```python
from build123d import *

# Parameters (mm, degrees)
F0_W     = 21.082
F0_H     = 12.7
F1_DEPTH = 5.08
F2_R     = 2.5019
F3_DEPTH = 5.08
F4_R     = 0.127


with BuildPart() as f1:
    # F0 (on Top) → F1 (new body)
    with BuildSketch(Plane.XY):
        Rectangle(F0_W, F0_H)
        with BuildLine():
            Line((-10.541, -6.35), (-10.541, 6.35))
            ThreePointArc((-10.541, 6.35), (-16.891, 0), (-10.541, -6.35))
        make_face()
        with BuildLine():
            ThreePointArc((10.541, -6.35), (16.891, 0), (10.541, 6.35))
            Line((10.541, 6.35), (10.541, -6.35))
        make_face()
    extrude(amount=F1_DEPTH)

    # F2 (on face) → F3 (join)
    with BuildSketch(Plane.XY.offset(5.08)):
        with Locations((-10.541, 0)):
            Circle(F2_R)
        with Locations((10.541, 0)):
            Circle(F2_R)
    extrude(amount=F3_DEPTH)

    # F4
    f4_edges = [f1.edges().sort_by_distance(p)[0] for p in [
        (-13.0429, 0, 10.16),
        (8.0391, 0, 10.16),
    ]]
    fillet(f4_edges, radius=F4_R)


solid = f1.part
```
Geometry check sheet. Reference: the model listing, model coordinates, mm. A direction names the side the tool comes from. Give positions to 0.01 mm unless a question says otherwise; leave off trailing zeros. Write each loop counter-clockwise with the first axis right and the second up, starting at its lowest first coordinate (ties: lowest second). Pieces come first, ordered by that corner, then holes. Notation, with made-up numbers: (40, -32.5) -> (69, -32.5) arc R9 cw to (69, -27.5) -> close; hole circle Ø10 at (76, 54). An arc over 180 degrees is marked (long way). Use one line per item in the form item = value.
Item 1: Sectioned sample at D-D on z = 2. Enter the section's corners in (x, y).
Results list:
outline = (-10.54, -6.35) -> (10.54, -6.35) arc R6.35 ccw to (10.54, 6.35) -> (-10.54, 6.35) arc R6.35 ccw to start
Item 2: Depth check by flat-ended pin: pin 1 Ø2 at (x, y) = (-4.5, -3) entering from +Z; pin 2 Ø1 at (y, z) = (5, 1) entering from -X. Enter the tip coordinate at first touch or a pass-through.
Results list:
pin_1 = 5.08
pin_2 = -15.02
Item 3: Access from +Z, -Z, +X, -X, +Y, -Y to the whole of each face (thin tool, end or side, straight path). Record for faces 1 (the cylindrical face through (8.04, 0.11, 7.52)), 2 (the flat face through (0, 0, 0)).
Results list:
face_1 = +Z
face_2 = -Z, +X, -X, +Y, -Y
Item 4: Mould release check, pull along X, two halves, no side actions. Record for faces 3 (the cylindrical face through (16.89, -0.14, 2.5)), 4 (the flat face through (0, 0, 5.08)), 5 (the cylindrical face through (-13.04, 0.11, 7.52)), 6 (the flat face through (0, 6.35, 3)): released by +X, released by -X, zero draft, split by the parting line, or undercut.
Results list:
face_3 = released by +X
face_4 = undercut
face_5 = undercut
face_6 = zero draft
Item 5: Sectioned sample at C-C on x = -5.5. Enter the section's corners in (y, z), plus the area to 3 significant figures.
Results list:
outline = (-6.35, 0) -> (6.35, 0) -> (6.35, 5.08) -> (-6.35, 5.08) -> close
area = 64.5 mm2
Item 6: Sectioned sample at A-A on y = 0. Enter the section's corners in (x, z), plus the area to 3 significant figures.
Results list:
outline = (-16.89, 0) -> (16.89, 0) -> (16.89, 5.08) -> (13.04, 5.08) -> (13.04, 10.03) arc R0.13 ccw to (12.92, 10.16) -> (8.17, 10.16) arc R0.13 ccw to (8.04, 10.03) -> (8.04, 5.08) -> (-8.04, 5.08) -> (-8.04, 10.03) arc R0.13 ccw to (-8.17, 10.16) -> (-12.92, 10.16) arc R0.13 ccw to (-13.04, 10.03) -> (-13.04, 5.08) -> (-16.89, 5.08) -> close
area = 222 mm2
Item 7: Scan lines: line 1 (Z direction, x = 1, y = 1.5); line 2 (X direction, y = 2.25, z = 8); line 3 (X direction, y = 1, z = 6.5). Record each from-to range of solid material in increasing order.
Results list:
line_1 = 0 to 5.08
line_2 = -11.64 to -9.45, 9.45 to 11.64
line_3 = -12.83 to -8.25, 8.25 to 12.83
Item 8: Sectioned sample at B-B on z = 8. Enter the section's corners in (x, y).
Results list:
outline = circle Ø5 at (-10.54, 0); circle Ø5 at (10.54, 0)
